```python
from build123d import *

# Parameters (mm, degrees)
F0_R     = 5
F1_DEPTH = 6


with BuildPart() as f1:
    # F0 (on Front) → F1 (new body)
    with BuildSketch(Plane.XZ):
        with BuildLine():
            Line((0, 130), (0, 0))
            Line((0, 0), (40, 0))
            Line((40, 0), (40, 40))
            ThreePointArc((40, 40), (36.262256, 52.252451), (35, 65))
            Line((35, 65), (35, 130))
            Line((35, 130), (0, 130))
        make_face()
        with Locations((20, 20)):
            Circle(F0_R, mode=Mode.SUBTRACT)
        with Locations((20, 50)):
            Circle(F0_R, mode=Mode.SUBTRACT)
        with Locations((20, 80)):
            Circle(F0_R, mode=Mode.SUBTRACT)
        with Locations((20, 110)):
            Circle(F0_R, mode=Mode.SUBTRACT)
    extrude(amount=F1_DEPTH)


solid = f1.part
```
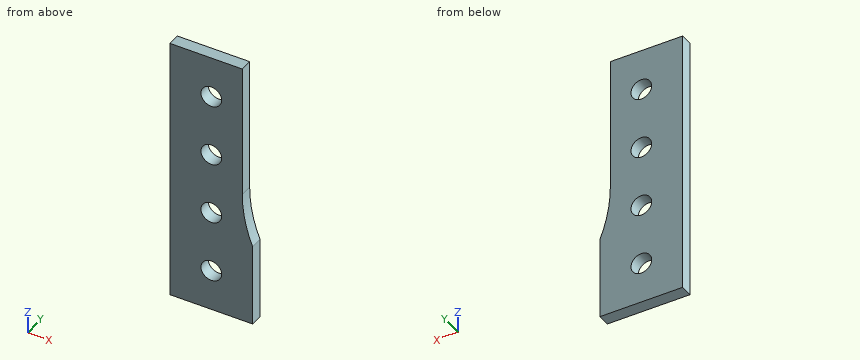
Work out the finished part from the listing and answer in its coordinate system (mm). Give positions to 0.01 mm unless a question says otherwise; leave off trailing zeros. Write each loop counter-clockwise with the first axis right and the second up, starting at its lowest first coordinate (ties: lowest second). Pieces come first, ordered by that corner, then holes. Notation, with made-up numbers: (82, 25) -> (101, 25) arc R31 cw to (101, 60) -> close; hole circle Ø5 at (62, 28.25). An arc over 180 degrees is marked (long way). Write each question's results on one line, items separated by ' | '.
1. Each of these flat-tipped pins is pushed along its axis until it touches: pin 1 Ø1.8 at (y, z) = (-3, 89) entering from +X; pin 2 Ø8 at (x, z) = (20, 20) entering from +Y. Where does it stop, or does it pass through?
Data:
pin 1: x = 35 | pin 2: through
2. Find section D-D on z = 110. Determine the outline of the cut face in (x, y).
Data:
outline: (0, -6) -> (15, -6) -> (15, 0) -> (0, 0) -> close; (25, -6) -> (35, -6) -> (35, 0) -> (25, 0) -> close
3. Find section C-C on x = 17. Determine the outline of the cut face in (y, z), and give its area (3 significant figures).
Data:
outline: (-6, 0) -> (0, 0) -> (0, 16) -> (-6, 16) -> close; (-6, 24) -> (0, 24) -> (0, 46) -> (-6, 46) -> close; (-6, 54) -> (0, 54) -> (0, 76) -> (-6, 76) -> close; (-6, 84) -> (0, 84) -> (0, 106) -> (-6, 106) -> close; (-6, 114) -> (0, 114) -> (0, 130) -> (-6, 130) -> close | area: 588 mm^2
4. Find section B-B on y = -4.4. Determine the outline of the cut face in (x, z), and give its area (3 significant figures).
Data:
outline: (0, 0) -> (40, 0) -> (40, 40) arc R65 cw to (35, 65) -> (35, 130) -> (0, 130) -> close; hole circle Ø10 at (20, 20); hole circle Ø10 at (20, 50); hole circle Ø10 at (20, 80); hole circle Ø10 at (20, 110) | area: 4,480 mm^2
5. Straight lines are drawn through the part: L1, parallel to Z at x = 20, y = -3.4; L2, parallel to Z at x = 17.5, y = -2.65; L3, parallel to X at y = -5.8, z = 73.5. For each, find the intervals that lie inside material, in ascending order.
Data:
L1: 0 to 15, 25 to 45, 55 to 75, 85 to 105, 115 to 130 | L2: 0 to 15.67, 24.33 to 45.67, 54.33 to 75.67, 84.33 to 105.67, 114.33 to 130 | L3: 0 to 35
6. Find section A-A on z = 20. Determine the outline of the cut face in (x, y).
Data:
outline: (0, -6) -> (15, -6) -> (15, 0) -> (0, 0) -> close; (25, -6) -> (40, -6) -> (40, 0) -> (25, 0) -> close
